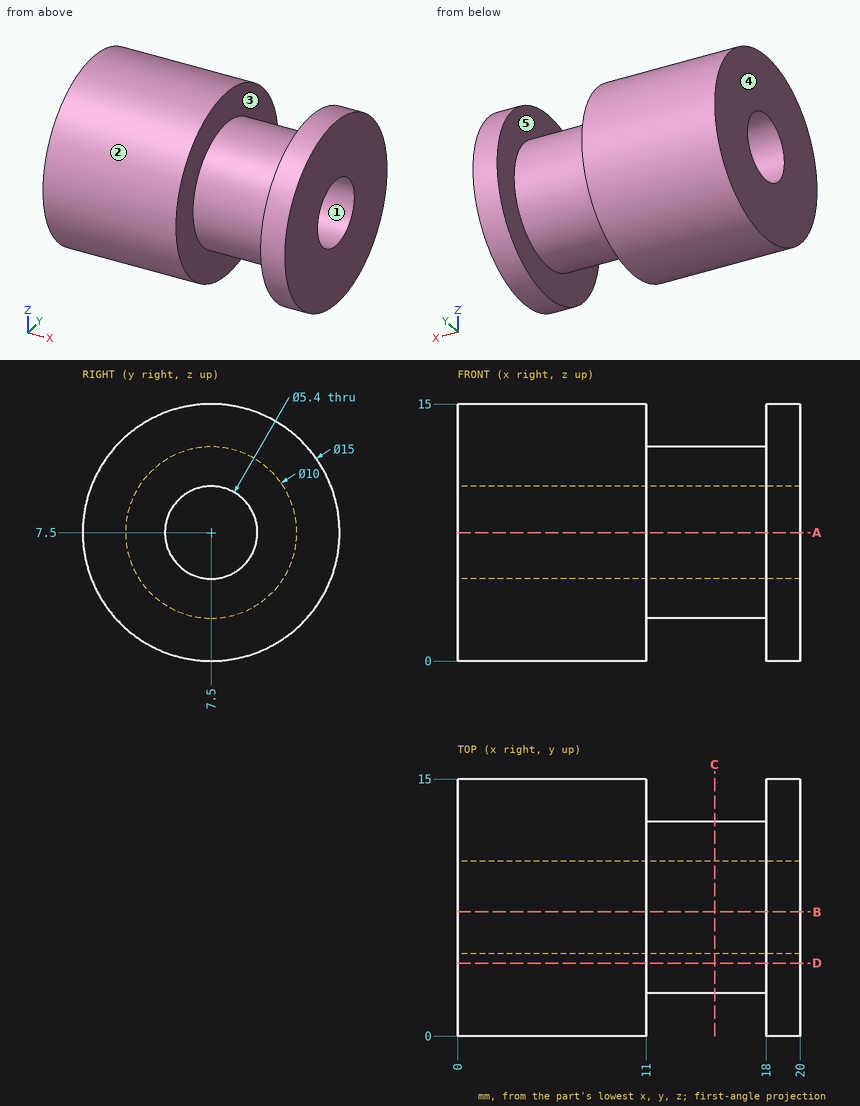
Input: dimensioned drawing with shaded views. Units: mm. Origin: part minimum x, y, z. A direction names the side the tool comes from. Give positions to 0.01 mm unless a question says otherwise; leave off trailing zeros. Write each loop counter-clockwise with the first axis right and the second up, starting at its lowest first coordinate (ties: lowest second). Pieces come first, ordered by that corner, then holes. Notation, with made-up numbers: M 22.5,-37 L 32.5,-37 A17 cw 32.5,-28 Z; hole C 51,61 d2. An arc over 180 degrees is marked long. Return JSON: item names as keys, results as strings. Group by question number.
1) Set-up query: the marked faces 4 and 5. Return all of +Z, -Z, +X, -X, +Y, -Y with unobstructed straight access to the full face (end or side cutting, diameter ignored); none if empty.
2) Pull-direction query (Y, two-part tool) for the marked faces 1, 2 and 3; classes: pulls with the +Y half, pulls with the -Y half, needs draft (parallel to the pull), parting line crosses it, or undercut.
3) Cut plane C-C, the plane x = 15. Output: boundary loops of the cut face in (y, z).
4) Material intervals for line 1 along Y through (x, z) = (15, 7.5); line 2 along X through (y, z) = (12, 11.25); line 3 along Y through (x, z) = (6, 7.5), sorted ascending. Write a range as [from, to].
5) Cut plane B-B, the plane y = 7.25. Output: boundary loops of the cut face in (x, z).
6) Pin query (flat end, axial travel): P1, Ø1, axis at x = 14.5, y = 5.5, coming from the +Z side; P2, Ø8, axis at x = 18, y = 12, coming from the +Z side; P3, Ø4, axis at x = 13.5, y = 6, coming from the -Z side. Return the tip coordinate at first contact, or that it passes through.
7) Cut plane A-A, the plane z = 7.5. Output: boundary loops of the cut face in (x, y).
8) Cut plane D-D, the plane y = 4.25. Output: boundary loops of the cut face in (x, z), plus the area to 3 significant figures.
Recorded:
{
 "1": {"face 4": "+Z, -Z, -X, +Y, -Y", "face 5": "none"},
 "2": {"face 1": "undercut", "face 2": "parting line crosses it", "face 3": "needs draft"},
 "3": {"outline": "C 7.5,7.5 d10; hole C 7.5,7.5 d5.4"},
 "4": {"line 1": "y = [2.5, 4.8], [10.2, 12.5]", "line 2": "x = [0, 11], [18, 20]", "line 3": "y = [0, 4.8], [10.2, 15]"},
 "5": {"outline": "M 0,0 L 11,0 L 11,2.51 L 18,2.51 L 18,0 L 20,0 L 20,4.81 L 0,4.81 Z; M 0,10.19 L 20,10.19 L 20,15 L 18,15 L 18,12.49 L 11,12.49 L 11,15 L 0,15 Z"},
 "6": {"P1": "stops at z = 12.27", "P2": "stops at z = 14.98", "P3": "stops at z = 2.5"},
 "7": {"outline": "M 0,0 L 11,0 L 11,2.5 L 18,2.5 L 18,0 L 20,0 L 20,4.8 L 0,4.8 Z; M 0,10.2 L 20,10.2 L 20,15 L 18,15 L 18,12.5 L 11,12.5 L 11,15 L 0,15 Z"},
 "8": {"outline": "M 0,0.74 L 11,0.74 L 11,3.7 L 18,3.7 L 18,0.74 L 20,0.74 L 20,14.26 L 18,14.26 L 18,11.3 L 11,11.3 L 11,14.26 L 0,14.26 Z", "area": "229 mm²"}
}
